```python
from build123d import *

# Parameters (mm, degrees)
SKETCH1_W           = 50
SKETCH1_H           = 50
BOSS_EXTRUDE1_DEPTH = 30
CUT_EXTRUDE1_REACH  = 48.368
SKETCH2_R           = 7.5
SKETCH4_W           = 20
SKETCH4_H           = 15
BOSS_EXTRUDE3_DEPTH = 30


with BuildPart() as part:
    # Sketch1 → Boss-Extrude1 (new body)
    with BuildSketch(Plane.XY):
        Rectangle(SKETCH1_W, SKETCH1_H)
    extrude(amount=BOSS_EXTRUDE1_DEPTH)

    # Sketch2 → Cut-Extrude1 (cut, up to next)
    with BuildSketch(Plane.XY.offset(30), mode=Mode.PRIVATE) as cut_extrude1_sk1:
        Circle(SKETCH2_R)
    cut_extrude1_tool1 = extrude(cut_extrude1_sk1.sketch, amount=-CUT_EXTRUDE1_REACH, mode=Mode.PRIVATE) & part.part
    add(cut_extrude1_tool1.solids().sort_by_distance((0, 0, 30))[0], mode=Mode.SUBTRACT)

    # Sketch4 → Boss-Extrude3 (add)
    with BuildSketch(Plane(origin=(0, 25, 0), x_dir=(1, 0, 0), z_dir=(0, 1, 0))):
        with Locations((-15, -7.5)):
            Rectangle(SKETCH4_W, SKETCH4_H)
    extrude(amount=BOSS_EXTRUDE3_DEPTH)


solid = part.part
```
Read the model definition and answer for the solid it produces. Units are mm, in the model's axes. A direction names the side the tool comes from. Give positions to 0.01 mm unless a question says otherwise; leave off trailing zeros. Loops run counter-clockwise (first coordinate to the right, second up) from the corner with the lowest first, then second, coordinate; pieces in that order, holes last.
Item 1: The mould has two halves that part along Y. Classify faces 1 (the flat face through (0, -25, 15)), 2 (the flat face through (-15, 55, 7)), 3 (the cylindrical face through (-7.493, 0.33, 15.21)), 4 (the flat face through (-15, 40, 15)): released by +Y, released by -Y, zero draft, split by the parting line, or undercut.
Item 2: The part is cut by section B-B (y = 0). Write down the section's boundary in (x, z).
Item 3: The part is cut by section A-A (z = 5). Write down the section's boundary in (x, y), and give its area (3 significant figures).
Item 4: Find the intervals of material crossed by line 1 along Y through (x, z) = (0, 11.75); line 2 along Y through (x, z) = (-21, 18.25); line 3 along X through (y, z) = (38, 13.5), in increasing order.
Item 5: The part is cut by section D-D (z = 24). Write down the section's boundary in (x, y).
Item 6: Each of these flat-tipped pins is pushed along its axis until it touches: pin 1 Ø10 at (x, y) = (-11.5, 36) entering from +Z; pin 2 Ø9 at (x, z) = (2.5, 20) entering from +Y; pin 3 Ø4.5 at (y, z) = (35.5, 10.5) entering from +X. Where does it stop, or does it pass through?
Item 7: For faces 5 (the flat face through (-6, 6, 30)), 6 (the flat face through (-5, 40, 8)), determine the directions among +Z, -Z, +X, -X, +Y, -Y from which every point of the face is accessible in a straight line to the end or side of a thin tool.
Taken from the geometry:
1. face 1: released by -Y
1. face 2: released by +Y
1. face 3: undercut
1. face 4: zero draft
2. outline: (-25, 0) - (-7.5, 0) - (-7.5, 30) - (-25, 30) - close; (7.5, 0) - (25, 0) - (25, 30) - (7.5, 30) - close
3. outline: (-25, -25) - (25, -25) - (25, 25) - (-5, 25) - (-5, 55) - (-25, 55) - close; hole circle Ø15 at (0, 0)
3. area: 2,920 mm2
4. line 1: y = -25 to -7.5, 7.5 to 25
4. line 2: y = -25 to 25
4. line 3: x = -25 to -5
5. outline: (-25, -25) - (25, -25) - (25, 25) - (-25, 25) - close; hole circle Ø15 at (0, 0)
6. pin 1: stops at z = 15
6. pin 2: stops at y = 25
6. pin 3: stops at x = -5
7. face 5: +Z, +X, -X, +Y, -Y
7. face 6: +Z, -Z, +X, +Y
